Design review of the part built by this model. Coordinates are the model's own, in mm. Face numbers are marked on the shaded views. A direction names the side the tool comes from. Round coordinates to 2 decimals unless told otherwise and drop trailing zeros. Order: outer loops, then holes, each group sorted by start corner. A loop starts at its lowest first (then second) coordinate and runs counter-clockwise, first axis right, second up. Notation, with made-up numbers: M -7.5,2.25 L -0.5,2.25 A24 cw -0.5,25.25 Z; hole C 44,-37 d1. An arc over 180 degrees is marked long. Use a Markdown table: item, result. Add a question column.
(1) To check wall thickness, follow probe 1 along Y at (x, z) = (0, 1) (3 decimals); probe 2 along Y at (x, z) = (-19.45, 9.25); probe 3 along Z at (x, y) = (9.5, -1.5). State the ranges of each line that lie inside material, in increasing order. Write a range as from..to.
(2) Take a section at D-D (z = 20.5). Write out the cut boundary in (x, y), then the cut area to 3 significant figures.
(3) Take a section at A-A (x = 0). Write out the cut boundary in (y, z) (3 decimals), then the cut area to 4 significant figures.
(4) For pin 1 (3 mm diameter, centred on x = -19, y = 0.5, fed in from -Z); pin 2 (5 mm diameter, centred on x = -10.75, y = 0, fed in from +Z); pin 3 (4 mm diameter, centred on x = -15, z = 7.5, fed in from -Y), all flat-tipped, find the tip position at first contact; note any pin that passes through.
(5) Take a section at C-C (x = -19.45). Write out the cut boundary in (y, z), then the cut area to 3 significant figures.
(6) Machinability: for the marked faces 4, 5 and 6, which of the approach directions +Z, -Z, +X, -X, +Y, -Y give a long, thin tool a straight path to every point of the face, cutting with its end or side? Answer none if there is none.
(7) Take a section at B-B (x = -10.75). Write out the cut boundary in (y, z), then the cut area to 3 significant figures.
(8) The part is to be moulded in two halves that separate along Z. For the marked faces 1, 2 and 3, say which applies: released by +Z, released by -Z, zero draft, split by the parting line, or undercut.
```python
from build123d import *

# Parameters (mm, degrees)
SKETCH1_R                = 1.5
SKETCH1_R_2              = 5
SKETCH1_R_3              = 3
BOSS_EXTRUDE1_DEPTH      = 3
SKETCH2_W                = 19.444746102
SKETCH2_H                = 10.693884422
SKETCH2_R                = 3
SKETCH2_R_2              = 1.5
BOSS_EXTRUDE2_DEPTH      = 3
BOSS_EXTRUDE3_DEPTH      = 28
BOSS_EXTRUDE3_DEPTH_BACK = 3
SKETCH3_R                = 3
SKETCH3_R_2              = 1.65
SKETCH4_R                = 0.5
CUT_EXTRUDE1_DEPTH       = 30
SKETCH5_R                = 3
CUT_EXTRUDE2_DEPTH       = 2
CHAMFER1_SIZE            = 1
FILLET2_R                = 1
FILLET3_R                = 1


with BuildPart() as part:
    # Sketch1 → Boss-Extrude1 (new body)
    # profile 1 of 4: a face of its own
    with BuildSketch(Plane.XY):
        with BuildLine():
            ThreePointArc((2.863548114, 10.119478732), (2.965690842, 9.677413339), (3, 9.225))
            ThreePointArc((3, 9.225), (-0.452413339, 6.259309158), (-2.863548114, 10.119478732))
            ThreePointArc((-2.863548114, 10.119478732), (-6.005253898, 5.346942211), (-11.199408085, 2.966147733))
            ThreePointArc((-11.199408085, 2.966147733), (-8.794012303, 2.274667476), (-7.75, 0))
            ThreePointArc((-7.75, 0), (-8.794012303, -2.274667476), (-11.199408085, -2.966147733))
            ThreePointArc((-11.199408085, -2.966147733), (-6.005253898, -5.346942211), (-2.863548114, -10.119478732))
            ThreePointArc((-2.863548114, -10.119478732), (0, -12.225), (2.863548114, -10.119478732))
            ThreePointArc((2.863548114, -10.119478732), (6.005253898, -5.346942211), (11.199408085, -2.966147733))
            ThreePointArc((11.199408085, -2.966147733), (7.75, 0), (11.199408085, 2.966147733))
            ThreePointArc((11.199408085, 2.966147733), (6.005253898, 5.346942211), (2.863548114, 10.119478732))
        make_face()
        with Locations((0, -9.225)):
            Circle(SKETCH1_R, mode=Mode.SUBTRACT)
        Circle(SKETCH1_R_2, mode=Mode.SUBTRACT)
    # profile 2 of 4: a face of its own
    with BuildSketch(Plane.XY):
        with Locations((0, 9.225)):
            Circle(SKETCH1_R_3)
        with Locations((0, 9.225)):
            Circle(SKETCH1_R, mode=Mode.SUBTRACT)
    # profile 3 of 4: a face of its own
    with BuildSketch(Plane.XY):
        with Locations((-10.75, 0)):
            Circle(SKETCH1_R_3)
        with Locations((-10.75, 0)):
            Circle(SKETCH1_R, mode=Mode.SUBTRACT)
    # profile 4 of 4: a face of its own
    with BuildSketch(Plane.XY):
        with Locations((10.75, 0)):
            Circle(SKETCH1_R_3)
        with Locations((10.75, 0)):
            Circle(SKETCH1_R, mode=Mode.SUBTRACT)
    extrude(amount=BOSS_EXTRUDE1_DEPTH)

    # Sketch2 → Boss-Extrude2 (add, through all)
    with BuildSketch(Plane(origin=(0, 0, 0), x_dir=(-1, 0, 0), z_dir=(0, 0, -1))):
        with Locations((15.727626949, 0)):
            Rectangle(SKETCH2_W, SKETCH2_H)
        with Locations((19.45, 0)):
            Circle(SKETCH2_R, mode=Mode.SUBTRACT)
        with Locations(Location((10.75, 0, 0), (0, 0, 180))):
            Circle(SKETCH2_R_2, mode=Mode.SUBTRACT)
    extrude(amount=-BOSS_EXTRUDE2_DEPTH)

    # Sketch3 → Boss-Extrude3 (add, two sides: drawn at the far end of the back side and taken through both)
    with BuildSketch(Plane.XY.offset(3).offset(-BOSS_EXTRUDE3_DEPTH_BACK)):
        with Locations((-19.45, 0)):
            Circle(SKETCH3_R)
        with Locations((-19.45, 0)):
            Circle(SKETCH3_R_2, mode=Mode.SUBTRACT)
    extrude(amount=BOSS_EXTRUDE3_DEPTH + BOSS_EXTRUDE3_DEPTH_BACK)

    # Sketch4 → Cut-Extrude1 (cut)
    with BuildSketch(Plane.XY.offset(31)):
        with Locations((-21.1, 0)):
            Circle(SKETCH4_R)
    extrude(amount=-CUT_EXTRUDE1_DEPTH, mode=Mode.SUBTRACT)

    # Sketch5 → Cut-Extrude2 (cut)
    with BuildSketch(Plane(origin=(0, 0, 0), x_dir=(-1, 0, 0), z_dir=(0, 0, -1))):
        with Locations(Location((19.45, 0, 0), (0, 0, 180))):
            Circle(SKETCH5_R)
    extrude(amount=-CUT_EXTRUDE2_DEPTH, mode=Mode.SUBTRACT)

    # Chamfer1
    # the kernel refuses this chamfer: 1 mm, written as the material it adds along each edge
    with BuildSketch(Plane(origin=(-19.45, 0, 2), x_dir=(1, 0, 0), z_dir=(0, 1, 0))) as chamfer1_piece_1_section:
        Polygon((3 - CHAMFER1_SIZE, 0), (3, CHAMFER1_SIZE), (3, 0), align=None)
    chamfer1_piece_1 = revolve(axis=Axis((-19.45, 0, 2), (0, 0, -1)), mode=Mode.PRIVATE)
    chamfer1_piece_1 = chamfer1_piece_1 - Plane(origin=(-21.1, 0, 1.51482841), x_dir=(1, 0, 0), z_dir=(0, 0, 1)) * Cylinder(0.5, 12, mode=Mode.PRIVATE)
    add(chamfer1_piece_1)

    # Fillet2
    fillet2_edges = [part.edges().sort_by_distance(p)[0] for p in [
        (-22.45, 0, 3),
    ]]
    fillet(fillet2_edges, radius=FILLET2_R)

    # Fillet3
    # the kernel refuses this fillet: 1 mm, written as the material it takes off along each edge
    with BuildSketch(Plane(origin=(-19.45, 0, 31), x_dir=(1, 0, 0), z_dir=(0, -1, 0))) as fillet3_piece_1:
        with BuildLine():
            CenterArc((3 - FILLET3_R, -FILLET3_R), FILLET3_R, 0, 90)
            Line((3 - FILLET3_R, 0), (3, 0))
            Line((3, 0), (3, -FILLET3_R))
        make_face()
    revolve(axis=Axis((-19.45, 0, 31), (0, 0, 1)), mode=Mode.SUBTRACT)


solid = part.part
```
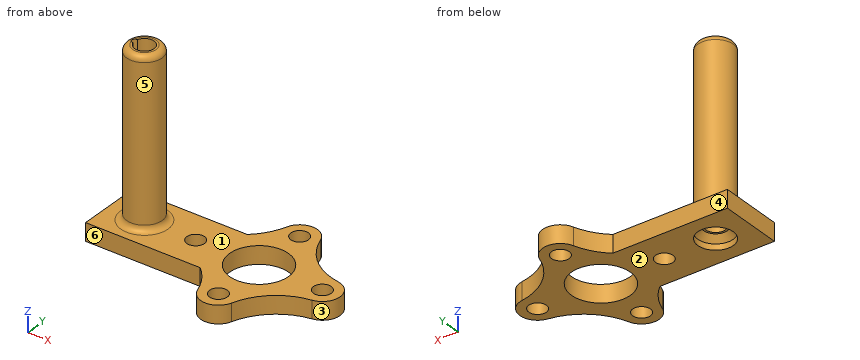
Verdict:
| question | item | result |
|---|---|---|
| 1 | probe 1 | y = -12.225..-10.725, -7.725..-5, 5..7.725, 10.725..12.225 |
| 1 | probe 2 | y = -3..-1.65, 1.65..3 |
| 1 | probe 3 | z = 0..3 |
| 2 | outline | C -19.45,0 d6; hole M -21.02,-0.49 A1.65 ccw long -21.02,0.49 A0.5 ccw long Z |
| 2 | area | 19.3 mm^2 |
| 3 | outline | M -12.225,0 L -10.725,0 L -10.725,3 L -12.225,3 Z; M -7.725,0 L -5,0 L -5,3 L -7.725,3 Z; M 5,0 L 7.725,0 L 7.725,3 L 5,3 Z; M 10.725,0 L 12.225,0 L 12.225,3 L 10.725,3 Z |
| 3 | area | 25.35 mm^2 |
| 4 | pin 1 | stops at z = 1.83 |
| 4 | pin 2 | stops at z = 3 |
| 4 | pin 3 | stops at y = -1.73 |
| 5 | outline | M -5.35,0 L -3,0 L -3,1 L -2,2 L -1.65,2 L -1.65,31 L -2,31 A1 ccw -3,30 L -3,4 A1 cw -4,3 L -5.35,3 Z; M 1.65,2 L 2,2 L 3,1 L 3,0 L 5.35,0 L 5.35,3 L 4,3 A1 cw 3,4 L 3,30 A1 ccw 2,31 L 1.65,31 Z |
| 5 | area | 93.4 mm^2 |
| 6 | face 4 | +Z, -Z, -X, +Y |
| 6 | face 5 | +Z |
| 6 | face 6 | +Z, -Z, -X, -Y |
| 7 | outline | M -5.35,0 L -1.5,0 L -1.5,3 L -5.35,3 Z; M 1.5,0 L 5.35,0 L 5.35,3 L 1.5,3 Z |
| 7 | area | 23.1 mm^2 |
| 8 | face 1 | released by +Z |
| 8 | face 2 | released by -Z |
| 8 | face 3 | zero draft |
